Here's how the part is built. I have some questions about the finished solid (model axes, mm). A direction names the side the tool comes from. Coordinates: 2 decimals unless noted, no trailing zeros. Loops run counter-clockwise (first coordinate to the right, second up) from the corner with the lowest first, then second, coordinate; pieces in that order, holes last. Notation, with made-up numbers: M 35,14 L 48,14 A13 cw 48,22 Z; hole C 70.25,-34.75 d6. An arc over 180 degrees is marked long. Use CSV: the item, a comma, the result in double quotes. Start each with the question number.
Q1. Please list where these lines run through material, in increasing order: probe 1 along X at (y, z) = (7, 24.25); probe 2 along Y at (x, z) = (3.75, 12.5). Write a range as [from, to].
Q2. If we section it at C-C (z = 12.5): Please give me the cut outline in (x, y), and give its area (3 significant figures).
Q3. If we mould it in two halves opening along Y, with no side actions, what happens to faces 1 (the flat face through (14, 8, 20)), 2 (the flat face through (8, 0, 12)), 3 (the flat face through (8, 16, 12))? For each: +Y half, -Y half, draft (parallel to the pull), parting line (faces both ways), or undercut.
Q4. Which directions (+Z, -Z, +X, -X, +Y, -Y) give clear straight access to the entire face, cutting with the end or side of a thin tool? Please do faces 4 (the flat face through (8, 14, 5)), 5 (the flat face through (8, 8, 15)), 6 (the cylindrical face through (8.11, 8.99, 12.63)).
Q5. For pin 1 Ø8 at (x, y) = (9.5, 8.5) entering from -Z, with a flat end and sliding along its axis, tell me the tip position at first contact or that it passes through.
Q6. If we section it at D-D (y = 5.5): Please give me the cut outline in (x, z).
Q7. If we section it at B-B (z = 8): Please give me the cut outline in (x, y).
Q8. If we section it at A-A (y = 8): Please give me the cut outline in (x, z).
from build123d import *

# Parameters (mm, degrees)
SKETCH_1_W          = 16
SKETCH_1_H          = 16
EXTRUDE_2_DEPTH     = 25
SKETCH_2_W          = 12
SKETCH_2_H          = 12
CUT_EXTRUDE_1_DEPTH = 10
SKETCH_4_W          = 12
SKETCH_4_H          = 12
CUT_EXTRUDE_3_DEPTH = 10
SKETCH_5_R          = 1
CUT_EXTRUDE_4_DEPTH = 18


with BuildPart() as part:
    # 草图1 → 凸台-拉伸2 (new body)
    with BuildSketch(Plane.XY):
        with Locations((8, 8)):
            Rectangle(SKETCH_1_W, SKETCH_1_H)
    extrude(amount=EXTRUDE_2_DEPTH)

    # 草图2 → 切除-拉伸1 (cut)
    with BuildSketch(Plane(origin=(0, 0, 0), x_dir=(-1, 0, 0), z_dir=(0, 0, -1))):
        with Locations((-8, 8)):
            Rectangle(SKETCH_2_W, SKETCH_2_H)
    extrude(amount=-CUT_EXTRUDE_1_DEPTH, mode=Mode.SUBTRACT)

    # 草图4 → 切除-拉伸3 (cut)
    with BuildSketch(Plane.XY.offset(25)):
        with Locations((8, 8)):
            Rectangle(SKETCH_4_W, SKETCH_4_H)
    extrude(amount=-CUT_EXTRUDE_3_DEPTH, mode=Mode.SUBTRACT)

    # 草图5 → 切除-拉伸4 (cut)
    with BuildSketch(Plane(origin=(16, 0, 0), x_dir=(0, 0, -1), z_dir=(1, 0, 0))):
        with Locations((-12.5, 8)):
            Circle(SKETCH_5_R)
    extrude(amount=-CUT_EXTRUDE_4_DEPTH, mode=Mode.SUBTRACT)


solid = part.part
Results below:
1,probe 1,"[0, 2], [14, 16]"
1,probe 2,"[0, 7], [9, 16]"
2,outline,"M 0,0 L 16,0 L 16,7 L 0,7 Z; M 0,9 L 16,9 L 16,16 L 0,16 Z"
2,area,"224 mm^2"
3,face 1,"undercut"
3,face 2,"-Y half"
3,face 3,"+Y half"
4,face 4,"-Z"
4,face 5,"+Z"
4,face 6,"+X, -X"
5,pin 1,"z = 10"
6,outline,"M 0,0 L 2,0 L 2,10 L 14,10 L 14,0 L 16,0 L 16,25 L 14,25 L 14,15 L 2,15 L 2,25 L 0,25 Z"
7,outline,"M 0,0 L 16,0 L 16,16 L 0,16 Z; hole M 2,2 L 14,2 L 14,14 L 2,14 Z"
8,outline,"M 0,0 L 2,0 L 2,10 L 14,10 L 14,0 L 16,0 L 16,11.5 L 0,11.5 Z; M 0,13.5 L 16,13.5 L 16,25 L 14,25 L 14,15 L 2,15 L 2,25 L 0,25 Z"
